```python
from build123d import *

# Parameters (mm, degrees)
SKETCH1_W             = 40
SKETCH1_H             = 30
BOSS_EXTRUDE1_DEPTH   = 6.35
SKETCH2_W             = 24.148
SKETCH2_H             = 6.858
CUT_EXTRUDE1_DEPTH    = 7.35
F_6_CLEARANCE_HOLE1_D = 3.6576


with BuildPart() as part:
    # Sketch1 → Boss-Extrude1 (new body)
    with BuildSketch(Plane(origin=(0, 0, 0), x_dir=(1, 0, 0), z_dir=(0, 1, 0))):
        Rectangle(SKETCH1_W, SKETCH1_H)
    extrude(amount=BOSS_EXTRUDE1_DEPTH)

    # Sketch2 → Cut-Extrude1 (cut, through all)
    with BuildSketch(Plane(origin=(0, 6.35, 0), x_dir=(1, 0, 0), z_dir=(0, 1, 0))):
        with Locations((0, 8.65)):
            Rectangle(SKETCH2_W, SKETCH2_H)
    extrude(amount=-CUT_EXTRUDE1_DEPTH, mode=Mode.SUBTRACT)

    # #6 Clearance Hole1 (through all)
    with Locations(Plane(origin=(0, 6.35, 0), x_dir=(1, 0, 0), z_dir=(0, 1, 0))):
        with Locations((0, -5.2438)):
            Hole(F_6_CLEARANCE_HOLE1_D / 2)


solid = part.part
```
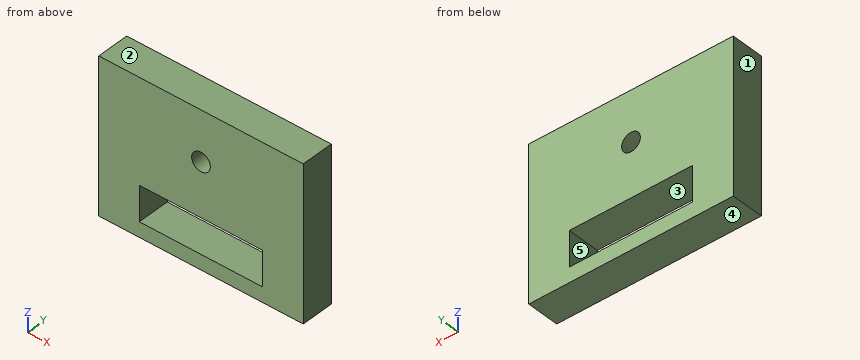
The listing builds one solid part. Answer for the finished solid, in the listing's coordinates (mm). Face numbers are marked on the shaded views. A direction names the side the tool comes from. Coordinates: 2 decimals unless noted, no trailing zeros. Order: outer loops, then holes, each group sorted by start corner. A loop starts at its lowest first (then second) coordinate and runs counter-clockwise, first axis right, second up. Notation, with made-up numbers: M 9.25,5.25 L 29.25,5.25 A31 ccw 29.25,44.25 Z; hole C -10.75,17 d1. An arc over 180 degrees is marked long. Answer as a JSON object with one key per item and string values. Group by question number.
1. Section A-A on x = 0 is taken. Write down the section's boundary in (y, z) (3 decimals), then the cut area to 3 significant figures.
2. Section B-B on x = -11 is taken. Write down the section's boundary in (y, z).
3. Determine the mould class of the marked faces 1, 2 and 3 for opening direction X: released by +X, released by -X, zero draft, split by the parting line, or undercut.
4. Straight lines are drawn through the part: line 1 (Z direction, x = 0, y = 1.75) (3 decimals); line 2 (X direction, y = 0.5, z = -10.5); line 3 (Z direction, x = 5, y = 2). For each, find the intervals that lie inside material, in ascending order.
5. A tool of negligible diameter and unlimited length cuts with its end or side. For the marked faces 4 and 5, from which of +Z, -Z, +X, -X, +Y, -Y can it reach the whole face along a straight path? Write none if from no direction.
6. Section C-C on y = 5 is taken. Write down the section's boundary in (x, z).
7. A flat-ended cylindrical pin translates along its axis: P1, Ø1.5, axis at x = 8.5, z = -10, coming from the -Y side. Find the tip coordinate at first contact, or state that the pin passes through.
Values follow:
{
 "1": {"outline": "M 0,-15 L 6.35,-15 L 6.35,-12.079 L 0,-12.079 Z; M 0,-5.221 L 6.35,-5.221 L 6.35,3.415 L 0,3.415 Z; M 0,7.073 L 6.35,7.073 L 6.35,15 L 0,15 Z", "area": "124 mm2"},
 "2": {"outline": "M 0,-15 L 6.35,-15 L 6.35,-12.08 L 0,-12.08 Z; M 0,-5.22 L 6.35,-5.22 L 6.35,15 L 0,15 Z"},
 "3": {"face 1": "released by -X", "face 2": "zero draft", "face 3": "undercut"},
 "4": {"line 1": "-15 to -12.079, -5.221 to 3.415, 7.073 to 15", "line 2": "-20 to -12.07, 12.07 to 20", "line 3": "-15 to -12.08, -5.22 to 15"},
 "5": {"face 4": "-Z, +X, -X, +Y, -Y", "face 5": "+Y, -Y"},
 "6": {"outline": "M -20,-15 L 20,-15 L 20,15 L -20,15 Z; hole M -12.07,-12.08 L 12.07,-12.08 L 12.07,-5.22 L -12.07,-5.22 Z; hole C 0,5.24 d3.66"},
 "7": {"P1": "through"}
}
